from build123d import *

# Parameters (mm, degrees)
SKETCH1_W           = 38
SKETCH1_H           = 47
BOSS_EXTRUDE1_DEPTH = 1.5
SKETCH2_R           = 3.25
CUT_EXTRUDE1_DEPTH  = 51.717354032
SKETCH3_R           = 2.425
CUT_EXTRUDE2_DEPTH  = 0.7
SKETCH4_R           = 2.425
BOSS_EXTRUDE2_DEPTH = 0.7
CHAMFER1_SIZE       = 1.5


with BuildPart() as part:
    # Sketch1 → Boss-Extrude1 (new body)
    with BuildSketch(Plane(origin=(0, 0, 0), x_dir=(0, 0, -1), z_dir=(1, 0, 0))):
        with Locations((0, 23.5)):
            Rectangle(SKETCH1_W, SKETCH1_H)
    extrude(amount=BOSS_EXTRUDE1_DEPTH)

    # Sketch2 → Cut-Extrude1 (cut, through all)
    with BuildSketch(Plane(origin=(1.5, 0, 0), x_dir=(0, 0, -1), z_dir=(1, 0, 0))):
        with Locations((0, 9)):
            Circle(SKETCH2_R)
        with Locations((0, 40)):
            Circle(SKETCH2_R)
    extrude(amount=-CUT_EXTRUDE1_DEPTH, mode=Mode.SUBTRACT)

    # Sketch3 → Cut-Extrude2 (cut)
    with BuildSketch(Plane.ZY):
        with Locations((-12, 40)):
            Circle(SKETCH3_R)
        with Locations((12, 40)):
            Circle(SKETCH3_R)
        with Locations((-12, 20.5)):
            Circle(SKETCH3_R)
        with Locations((12, 20.5)):
            Circle(SKETCH3_R)
    extrude(amount=-CUT_EXTRUDE2_DEPTH, mode=Mode.SUBTRACT)

    # Sketch4 → Boss-Extrude2 (add)
    with BuildSketch(Plane(origin=(1.5, 0, 0), x_dir=(0, 0, -1), z_dir=(1, 0, 0))):
        with Locations(Location((-12, 40, 0), (0, 0, 180))):
            Circle(SKETCH4_R)
        with Locations(Location((12, 40, 0), (0, 0, 180))):
            Circle(SKETCH4_R)
        with Locations(Location((-12, 20.5, 0), (0, 0, 180))):
            Circle(SKETCH4_R)
        with Locations(Location((12, 20.5, 0), (0, 0, 180))):
            Circle(SKETCH4_R)
    extrude(amount=BOSS_EXTRUDE2_DEPTH)

    # Chamfer1
    chamfer1_edges = [part.edges().sort_by_distance(p)[0] for p in [
        (0.75, 0, -19),
        (0.75, 0, 19),
    ]]
    chamfer(chamfer1_edges, length=CHAMFER1_SIZE)


solid = part.part
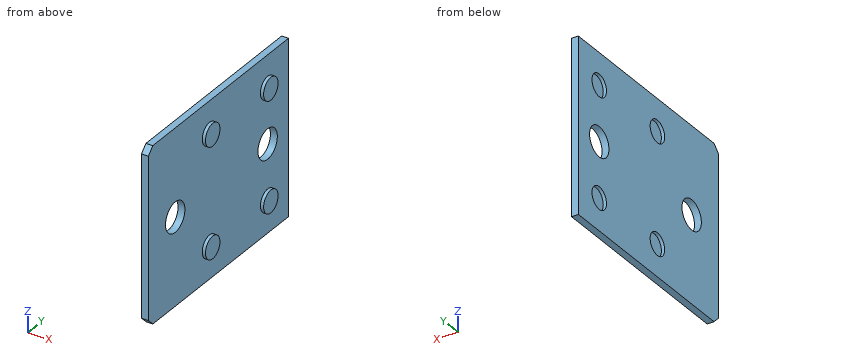
For this review, take the finished solid that the model builds, in its own axes (mm). Round coordinates to 2 decimals unless told otherwise and drop trailing zeros. Loops run counter-clockwise (first coordinate to the right, second up) from the corner with the lowest first, then second, coordinate; pieces in that order, holes last. Notation, with made-up numbers: (40, 25) - (81, 25) arc R15 cw to (81, 53) - close; hole circle Ø10 at (83, -14). An arc over 180 degrees is marked (long way). Put each result on its own line as item: value. Start each with the question number.
1. Consider section A-A on y = 9. State the section outline as (x, z) points, plus the area to 4 significant figures.
2. Insertion check: P1, Ø8.5, axis at y = 9, z = 0, coming from the +X side; P2, Ø1.5, axis at y = 39, z = 12.5, coming from the -X side. Each pin has a flat end and moves straight along its axis. Give the tip position at first contact, or say it passes through.
3. Consider section B-B on z = 0. State the section outline as (x, y) points, plus the area to 3 significant figures.
4. For probe 1 along Y at (x, z) = (0.4, 12) (3 decimals); probe 2 along Y at (x, z) = (0.65, 0); probe 3 along X at (y, z) = (8, 7), list the stretches that pass through material, from the lowest coordinate up. Write a range as [from, to].
5. Consider section D-D on z = -12. State the section outline as (x, y) points (3 decimals).
6. Consider section C-C on x = 1.15. State the section outline as (y, z) points, plus the area to 3 significant figures.
Result sheet:
1. outline: (0, -19) - (1.5, -19) - (1.5, -3.25) - (0, -3.25) - close; (0, 3.25) - (1.5, 3.25) - (1.5, 19) - (0, 19) - close
1. area: 47.25 mm^2
2. P1: x = 1.5
2. P2: x = 0.7
3. outline: (0, 0) - (1.5, 0) - (1.5, 5.75) - (0, 5.75) - close; (0, 12.25) - (1.5, 12.25) - (1.5, 36.75) - (0, 36.75) - close; (0, 43.25) - (1.5, 43.25) - (1.5, 47) - (0, 47) - close
3. area: 51.0 mm^2
4. probe 1: [0, 18.075], [22.925, 37.575], [42.425, 47]
4. probe 2: [0, 5.75], [12.25, 36.75], [43.25, 47]
4. probe 3: [0, 1.5]
5. outline: (0, 0) - (1.5, 0) - (1.5, 18.075) - (2.2, 18.075) - (2.2, 22.925) - (1.5, 22.925) - (1.5, 37.575) - (2.2, 37.575) - (2.2, 42.425) - (1.5, 42.425) - (1.5, 47) - (0, 47) - (0, 42.425) - (0.7, 42.425) - (0.7, 37.575) - (0, 37.575) - (0, 22.925) - (0.7, 22.925) - (0.7, 18.075) - (0, 18.075) - close
6. outline: (0, -17.5) - (1.5, -19) - (47, -19) - (47, 19) - (1.5, 19) - (0, 17.5) - close; hole circle Ø6.5 at (9, 0); hole circle Ø6.5 at (40, 0)
6. area: 1,720 mm^2
